Design review of the part shown in the three views and the two pictorial views. Dimensions are in mm from the part's minimum x, y and z. A direction names the side the tool comes from. Coordinates: 2 decimals unless noted, no trailing zeros. Loops run counter-clockwise (first coordinate to the right, second up) from the corner with the lowest first, then second, coordinate; pieces in that order, holes last.
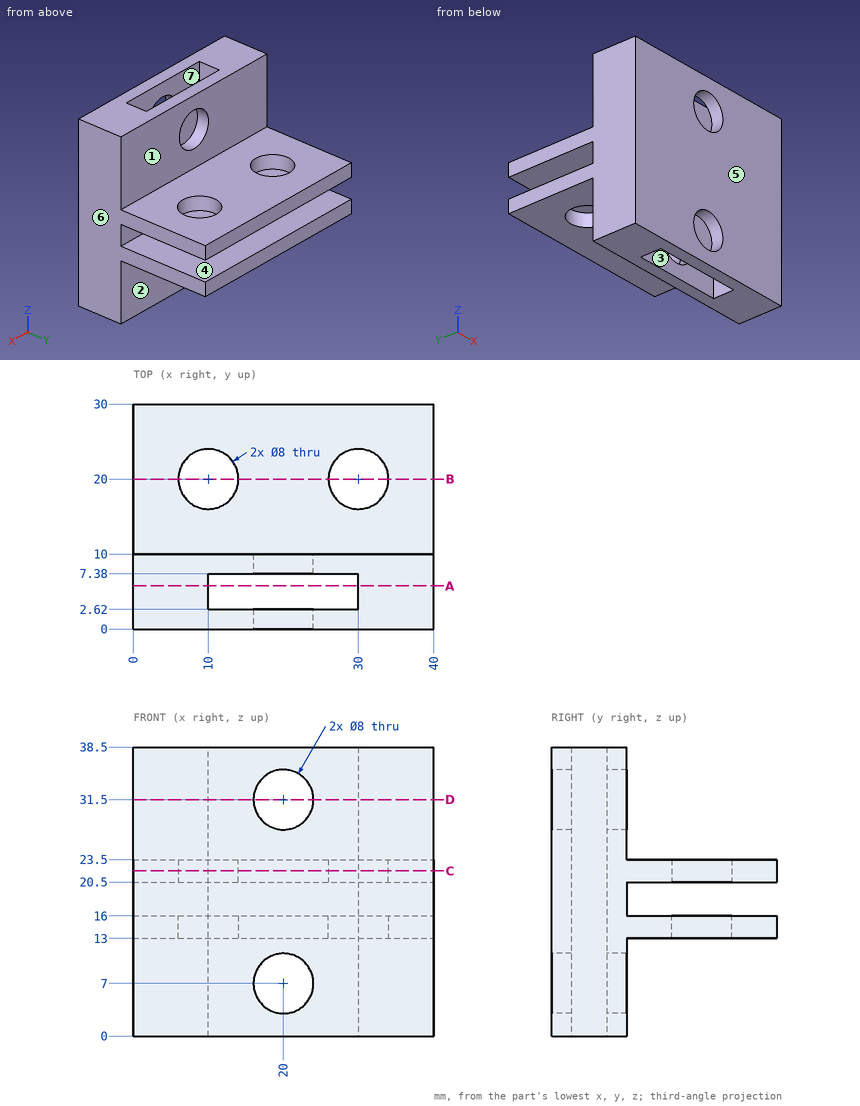
Q1. Consider section D-D (z = 31.5). State the section outline as (x, y) points, then the cut area to 3 significant figures.
Q2. Consider section B-B (y = 20). State the section outline as (x, z) points.
Q3. For pin 1 Ø4 at (x, y) = (16, 26) entering from -Z; pin 2 Ø10.5 at (x, z) = (20, 7) entering from +Y; pin 3 Ø9 at (x, y) = (30, 20) entering from +Z, all flat-tipped, find the tip position at first contact; note any pin that passes through.
Q4. The part is to be moulded in two halves that separate along X. For the marked faces 5, 6 and 7, say which applies: +X half, -X half, draft (parallel to the pull), parting line (faces both ways), or undercut.
Q5. Wall thickness on probe 1 along Z at (x, y) = (20, 1.3); probe 2 along Y at (x, z) = (11, 2.5); probe 3 along X at (y, z) = (6, 32.5): over which ranges is each line inside the solid? List them lowest first.
Q6. Machinability: for the marked faces 1, 2, 3 and 4, which of the approach directions +Z, -Z, +X, -X, +Y, -Y give a long, thin tool a straight path to every point of the face, cutting with its end or side? Answer none if there is none.
Q7. Consider section C-C (z = 22). State the section outline as (x, y) points, then the cut area to 3 significant figures.
Q8. Consider section A-A (y = 5.75). State the section outline as (x, z) points, then the cut area to 3 significant figures.
Model answer:
1. outline: (0, 0) - (16, 0) - (16, 2.62) - (10, 2.62) - (10, 7.38) - (16, 7.38) - (16, 10) - (0, 10) - close; (24, 0) - (40, 0) - (40, 10) - (24, 10) - (24, 7.38) - (30, 7.38) - (30, 2.62) - (24, 2.62) - close
1. area: 263 mm2
2. outline: (0, 13) - (6, 13) - (6, 16) - (0, 16) - close; (0, 20.5) - (6, 20.5) - (6, 23.5) - (0, 23.5) - close; (14, 13) - (26, 13) - (26, 16) - (14, 16) - close; (14, 20.5) - (26, 20.5) - (26, 23.5) - (14, 23.5) - close; (34, 13) - (40, 13) - (40, 16) - (34, 16) - close; (34, 20.5) - (40, 20.5) - (40, 23.5) - (34, 23.5) - close
3. pin 1: stops at z = 13
3. pin 2: stops at y = 10
3. pin 3: stops at z = 23.5
4. face 5: draft
4. face 6: +X half
4. face 7: undercut
5. probe 1: z = 0 to 3, 11 to 27.5, 35.5 to 38.5
5. probe 2: y = 0 to 2.62, 7.38 to 10
5. probe 3: x = 0 to 10, 30 to 40
6. face 1: +Z, +X, -X, +Y
6. face 2: -Z, +X, -X, +Y
6. face 3: +Z, -Z
6. face 4: +X, -X, +Y
7. outline: (0, 0) - (40, 0) - (40, 30) - (0, 30) - close; hole circle Ø8 at (10, 20); hole (10, 2.62) - (30, 2.62) - (30, 7.38) - (10, 7.38) - close; hole circle Ø8 at (30, 20)
7. area: 1,000 mm2
8. outline: (0, 0) - (10, 0) - (10, 38.5) - (0, 38.5) - close; (30, 0) - (40, 0) - (40, 38.5) - (30, 38.5) - close
8. area: 770 mm2
